Geometry: see drawing. Coordinates: mm, zero at the bounding-box minimum. A direction names the side the tool comes from. Round coordinates to 2 decimals unless told otherwise and drop trailing zeros. Loops run counter-clockwise (first coordinate to the right, second up) from the corner with the lowest first, then second, coordinate; pieces in that order, holes last. Notation, with made-up numbers: (-37, -25) -> (8, -25) arc R10 cw to (8, -12) -> close; hole circle Ø8 at (67, -8). An arc over 180 degrees is marked (long way). Answer in a Markdown table with one row per item.
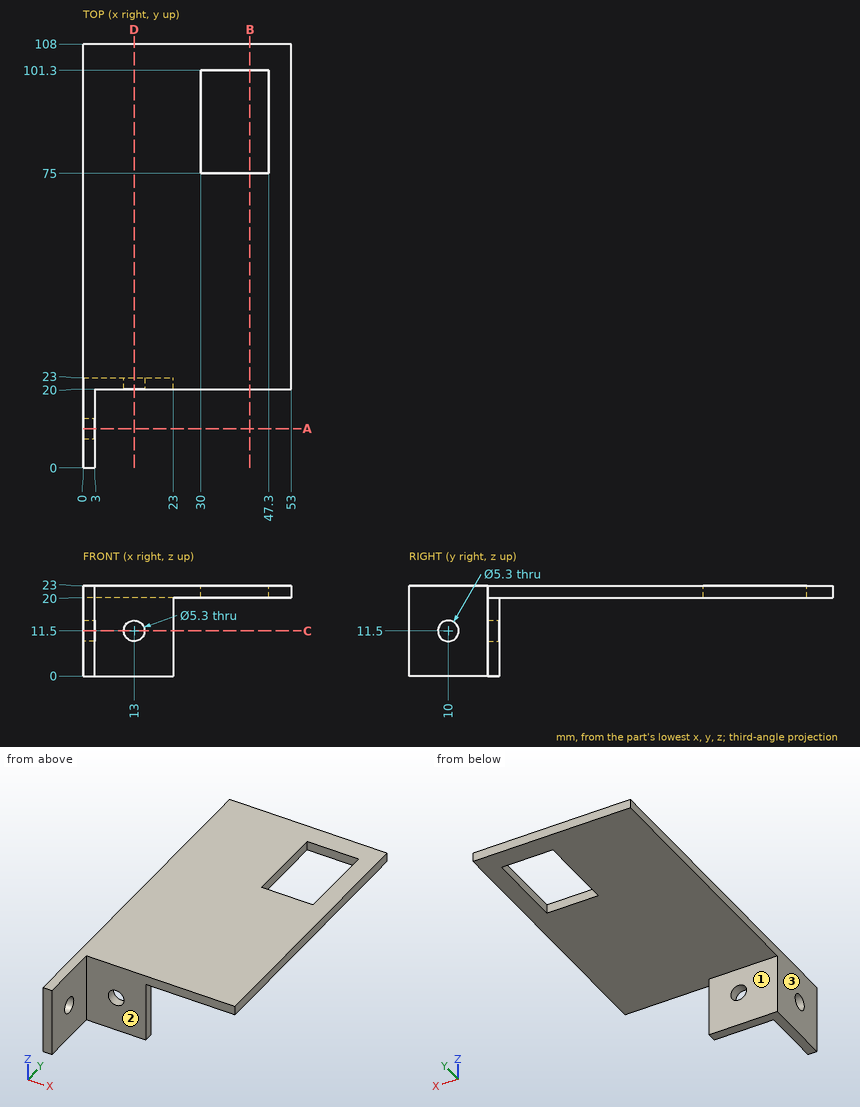
Item 1: Section query B-B, the plane x = 42.5. Output: boundary loops of the cut face in (y, z).
Ans:
| item | result |
|---|---|
| outline | (20, 20) -> (75, 20) -> (75, 23) -> (20, 23) -> close; (101.3, 20) -> (108, 20) -> (108, 23) -> (101.3, 23) -> close |
Item 2: Section query C-C, the plane z = 11.5. Output: boundary loops of the cut face in (x, y), and give its area (3 significant figures).
Ans:
| item | result |
|---|---|
| outline | (0, 0) -> (3, 0) -> (3, 7.35) -> (0, 7.35) -> close; (0, 12.65) -> (3, 12.65) -> (3, 20) -> (10.35, 20) -> (10.35, 23) -> (0, 23) -> close; (15.65, 20) -> (23, 20) -> (23, 23) -> (15.65, 23) -> close |
| area | 97.2 mm2 |
Item 3: Set-up query: the marked faces 1, 2 and 3. Return all of +Z, -Z, +X, -X, +Y, -Y with unobstructed straight access to the full face (end or side cutting, diameter ignored); none if empty.
Ans:
| item | result |
|---|---|
| face 1 | -Z, +X, -X, +Y |
| face 2 | +Z, -Z, +X, -Y |
| face 3 | +Z, -Z, -X, +Y, -Y |
Item 4: First-contact query: P1, Ø8.5, axis at x = 13, z = 11.5, coming from the +Y side; P2, Ø10, axis at x = 15.5, z = 14.5, coming from the -Y side; P3, Ø1.5, axis at y = 21, z = 7.5, coming from the +X side; P4, Ø4, axis at y = 26, z = 3, coming from the -X side. Flat tips, straight axial feed; report the tip coordinate or a pass-through.
Ans:
| item | result |
|---|---|
| P1 | y = 23 |
| P2 | y = 20 |
| P3 | x = 23 |
| P4 | through |
Item 5: Section query D-D, the plane x = 13. Output: boundary loops of the cut face in (y, z).
Ans:
| item | result |
|---|---|
| outline | (20, 0) -> (23, 0) -> (23, 8.85) -> (20, 8.85) -> close; (20, 14.15) -> (23, 14.15) -> (23, 20) -> (108, 20) -> (108, 23) -> (20, 23) -> close |
Item 6: Section query A-A, the plane y = 10. Output: boundary loops of the cut face in (x, z), and give its area (3 significant figures).
Ans:
| item | result |
|---|---|
| outline | (0, 0) -> (3, 0) -> (3, 8.85) -> (0, 8.85) -> close; (0, 14.15) -> (3, 14.15) -> (3, 23) -> (0, 23) -> close |
| area | 53.1 mm2 |
Item 7: Ray query, L1, parallel to Y at x = 2.25, z = 11.5; L2, parallel to X at y = 21.8, z = 11.5; L3, parallel to Y at x = 31.5, z = 21.25. Return the intervals inside material, ascending.
Ans:
| item | result |
|---|---|
| L1 | 0 to 7.35, 12.65 to 23 |
| L2 | 0 to 10.35, 15.65 to 23 |
| L3 | 20 to 75, 101.3 to 108 |
